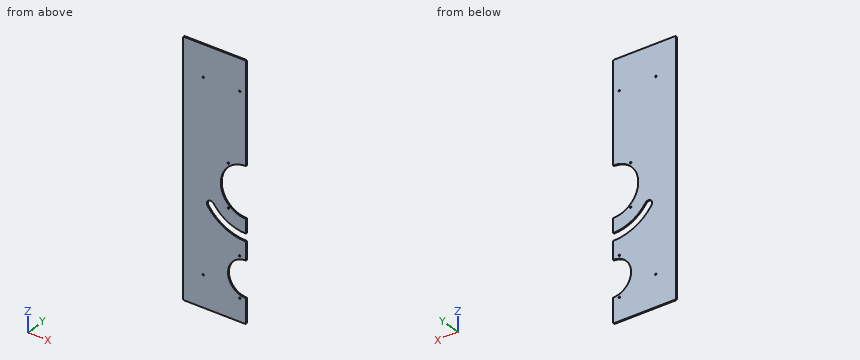
```python
from build123d import *

# Parameters (mm, degrees)
SKETCH1_W           = 250
SKETCH1_H           = 1000
BOSS_EXTRUDE1_DEPTH = 5
FILLET1_R           = 3
CUT_EXTRUDE2_REACH  = 7
SKETCH3_R           = 71.5
SKETCH3_R_2         = 100
SKETCH3_R_3         = 3


with BuildPart() as part:
    # Sketch1 → Boss-Extrude1 (new body)
    with BuildSketch(Plane(origin=(0, 0, 0), x_dir=(1, 0, 0), z_dir=(0, 1, 0))):
        Rectangle(SKETCH1_W, SKETCH1_H)
    extrude(amount=BOSS_EXTRUDE1_DEPTH)

    # Fillet1
    fillet1_edges = [part.edges().sort_by_distance(p)[0] for p in [
        (125, 2.5, 500),
        (-125, 2.5, 500),
        (-125, 2.5, -500),
        (125, 2.5, -500),
    ]]
    fillet(fillet1_edges, radius=FILLET1_R)

    # Sketch3 → Cut-Extrude2 (cut, up to next)
    with BuildSketch(Plane(origin=(0, 5, 0), x_dir=(1, 0, 0), z_dir=(0, 1, 0)), mode=Mode.PRIVATE) as cut_extrude2_sk1:
        with Locations((125, 330)):
            Circle(SKETCH3_R)
    cut_extrude2_tool1 = extrude(cut_extrude2_sk1.sketch, amount=-CUT_EXTRUDE2_REACH, mode=Mode.PRIVATE) & part.part
    add(cut_extrude2_tool1.solids().sort_by_distance((125, 5, -330))[0], mode=Mode.SUBTRACT)
    # Sketch3 → Cut-Extrude2 (cut, up to next)
    with BuildSketch(Plane(origin=(0, 5, 0), x_dir=(1, 0, 0), z_dir=(0, 1, 0)), mode=Mode.PRIVATE) as cut_extrude2_sk2:
        with Locations((125, 0)):
            Circle(SKETCH3_R_2)
    cut_extrude2_tool2 = extrude(cut_extrude2_sk2.sketch, amount=-CUT_EXTRUDE2_REACH, mode=Mode.PRIVATE) & part.part
    add(cut_extrude2_tool2.solids().sort_by_distance((125, 5, 0))[0], mode=Mode.SUBTRACT)
    # Sketch3 → Cut-Extrude2 (cut, up to next)
    with BuildSketch(Plane(origin=(0, 5, 0), x_dir=(1, 0, 0), z_dir=(0, 1, 0)), mode=Mode.PRIVATE) as cut_extrude2_sk3:
        with Locations((-45, -375)):
            Circle(SKETCH3_R_3)
    cut_extrude2_tool3 = extrude(cut_extrude2_sk3.sketch, amount=-CUT_EXTRUDE2_REACH, mode=Mode.PRIVATE) & part.part
    add(cut_extrude2_tool3.solids().sort_by_distance((-45, 5, 375))[0], mode=Mode.SUBTRACT)
    # Sketch3 → Cut-Extrude2 (cut, up to next)
    with BuildSketch(Plane(origin=(0, 5, 0), x_dir=(1, 0, 0), z_dir=(0, 1, 0)), mode=Mode.PRIVATE) as cut_extrude2_sk4:
        with Locations((-45, 375)):
            Circle(SKETCH3_R_3)
    cut_extrude2_tool4 = extrude(cut_extrude2_sk4.sketch, amount=-CUT_EXTRUDE2_REACH, mode=Mode.PRIVATE) & part.part
    add(cut_extrude2_tool4.solids().sort_by_distance((-45, 5, -375))[0], mode=Mode.SUBTRACT)
    # Sketch3 → Cut-Extrude2 (cut, up to next)
    with BuildSketch(Plane(origin=(0, 5, 0), x_dir=(1, 0, 0), z_dir=(0, 1, 0)), mode=Mode.PRIVATE) as cut_extrude2_sk5:
        with Locations((55, -85)):
            Circle(SKETCH3_R_3)
    cut_extrude2_tool5 = extrude(cut_extrude2_sk5.sketch, amount=-CUT_EXTRUDE2_REACH, mode=Mode.PRIVATE) & part.part
    add(cut_extrude2_tool5.solids().sort_by_distance((55, 5, 85))[0], mode=Mode.SUBTRACT)
    # Sketch3 → Cut-Extrude2 (cut, up to next)
    with BuildSketch(Plane(origin=(0, 5, 0), x_dir=(1, 0, 0), z_dir=(0, 1, 0)), mode=Mode.PRIVATE) as cut_extrude2_sk6:
        with Locations((55, 85)):
            Circle(SKETCH3_R_3)
    cut_extrude2_tool6 = extrude(cut_extrude2_sk6.sketch, amount=-CUT_EXTRUDE2_REACH, mode=Mode.PRIVATE) & part.part
    add(cut_extrude2_tool6.solids().sort_by_distance((55, 5, -85))[0], mode=Mode.SUBTRACT)
    # Sketch3 → Cut-Extrude2 (cut, up to next)
    with BuildSketch(Plane(origin=(0, 5, 0), x_dir=(1, 0, 0), z_dir=(0, 1, 0)), mode=Mode.PRIVATE) as cut_extrude2_sk7:
        with Locations((100, 410)):
            Circle(SKETCH3_R_3)
    cut_extrude2_tool7 = extrude(cut_extrude2_sk7.sketch, amount=-CUT_EXTRUDE2_REACH, mode=Mode.PRIVATE) & part.part
    add(cut_extrude2_tool7.solids().sort_by_distance((100, 5, -410))[0], mode=Mode.SUBTRACT)
    # Sketch3 → Cut-Extrude2 (cut, up to next)
    with BuildSketch(Plane(origin=(0, 5, 0), x_dir=(1, 0, 0), z_dir=(0, 1, 0)), mode=Mode.PRIVATE) as cut_extrude2_sk8:
        with Locations((100, 250)):
            Circle(SKETCH3_R_3)
    cut_extrude2_tool8 = extrude(cut_extrude2_sk8.sketch, amount=-CUT_EXTRUDE2_REACH, mode=Mode.PRIVATE) & part.part
    add(cut_extrude2_tool8.solids().sort_by_distance((100, 5, -250))[0], mode=Mode.SUBTRACT)
    # Sketch3 → Cut-Extrude2 (cut, up to next)
    with BuildSketch(Plane(origin=(0, 5, 0), x_dir=(1, 0, 0), z_dir=(0, 1, 0)), mode=Mode.PRIVATE) as cut_extrude2_sk9:
        with Locations((100, -375)):
            Circle(SKETCH3_R_3)
    cut_extrude2_tool9 = extrude(cut_extrude2_sk9.sketch, amount=-CUT_EXTRUDE2_REACH, mode=Mode.PRIVATE) & part.part
    add(cut_extrude2_tool9.solids().sort_by_distance((100, 5, 375))[0], mode=Mode.SUBTRACT)
    # Sketch3 → Cut-Extrude2 (cut, up to next)
    with BuildSketch(Plane(origin=(0, 5, 0), x_dir=(1, 0, 0), z_dir=(0, 1, 0)), mode=Mode.PRIVATE) as cut_extrude2_sk10:
        with BuildLine():
            ThreePointArc((125, 186.5), (38.883883632, 165.427520388), (-27.77185626, 106.972005379))
            ThreePointArc((-27.77185626, 106.972005379), (-24.088222141, 86.08107817), (-3.197294931, 89.764712289))
            ThreePointArc((-3.197294931, 89.764712289), (52.736342029, 138.817195392), (125, 156.5))
            ThreePointArc((125, 156.5), (140, 171.5), (125, 186.5))
        make_face()
    cut_extrude2_tool10 = extrude(cut_extrude2_sk10.sketch, amount=-CUT_EXTRUDE2_REACH, mode=Mode.PRIVATE) & part.part
    add(cut_extrude2_tool10.solids().sort_by_distance((49.559691, 5, -144.919486))[0], mode=Mode.SUBTRACT)


solid = part.part
```
Can you work these out from the model? Positions are in its coordinate system, mm. Round coordinates to 2 decimals unless told otherwise and drop trailing zeros. Loops run counter-clockwise (first coordinate to the right, second up) from the corner with the lowest first, then second, coordinate; pieces in that order, holes last. Notation, with made-up numbers: M 30.5,-37.75 L 48.5,-37.75 A37 cw 48.5,-0.75 Z; hole C -27,79.25 d9. An arc over 180 degrees is marked long. Answer as a JSON object with one key per item and string values. Group by question number.
Q1. Imagine slicing it at A-A, the plane y = 0.85. Please give me the cut outline in (x, z), then the cut area to 3 significant figures.
Q2. Please list where these lines run through material, in increasing order: L1, parallel to X at y = 3.45, z = 375; L2, parallel to Z at x = 46, y = 2; L3, parallel to Z at x = 35, y = 0.55.
Q3. Imagine slicing it at B-B, the plane z = 0. Please give me the cut outline in (x, y), then the cut area to 3 significant figures.
Findings:
{
 "1": {"outline": "M -125,-497 A3 ccw -122,-500 L 122,-500 A3 ccw 125,-497 L 125,-401.5 A71.5 cw 125,-258.5 L 125,-186.5 A186.5 cw -27.77,-106.97 A15 cw -3.2,-89.76 A156.5 ccw 125,-156.5 L 125,-100 A100 cw 125,100 L 125,497 A3 ccw 122,500 L -122,500 A3 ccw -125,497 Z; hole C -45,-375 d6; hole C -45,375 d6; hole C 55,-85 d6; hole C 55,85 d6; hole C 100,-410 d6; hole C 100,-250 d6; hole C 100,375 d6", "area": "221,000 mm2"},
 "2": {"L1": "x = -125 to -48, -42 to 97, 103 to 125", "L2": "z = -500 to -168.94, -135.1 to -61.31, 61.31 to 500", "L3": "z = -500 to -163.35, -128.03 to -43.59, 43.59 to 500"},
 "3": {"outline": "M -125,0 L 25,0 L 25,5 L -125,5 Z", "area": "750 mm2"}
}
